```python
from build123d import *

# Parameters (mm, degrees)
SKETCH004_W  = 65.024
SKETCH004_H  = 49.2125
PAD004_DEPTH = 2.54
SKETCH005_W  = 49.341553
SKETCH005_H  = 34.925
PAD005_DEPTH = 2.54


with BuildPart() as inverterlowerbracket:
    # Sketch004 → Pad004 (new body)
    with BuildSketch(Plane.YZ):
        with Locations((-55.960957, 1378.268994)):
            Rectangle(SKETCH004_W, SKETCH004_H)
        with BuildLine():
            ThreePointArc((-82.122957, 1396.525244), (-85.297957, 1393.350244), (-82.122957, 1390.175244))
            Line((-82.122957, 1390.175244), (-59.897957, 1390.175244))
            ThreePointArc((-59.897957, 1390.175244), (-56.722957, 1393.350244), (-59.897957, 1396.525244))
            Line((-82.122957, 1396.525244), (-59.897957, 1396.525244))
        make_face(mode=Mode.SUBTRACT)
        with BuildLine():
            ThreePointArc((-82.122957, 1366.362744), (-85.297957, 1363.187744), (-82.122957, 1360.012744))
            Line((-82.122957, 1360.012744), (-59.897957, 1360.012744))
            ThreePointArc((-59.897957, 1360.012744), (-56.722957, 1363.187744), (-59.897957, 1366.362744))
            Line((-82.122957, 1366.362744), (-59.897957, 1366.362744))
        make_face(mode=Mode.SUBTRACT)
    extrude(amount=PAD004_DEPTH)

    # Sketch005 (on Face1 of Pad004) → Pad005 (join)
    with BuildSketch(Plane.ZX.offset(-23.448957)):
        with Locations((1378.334228, -14.922899)):
            Rectangle(SKETCH005_W, SKETCH005_H)
        with BuildLine():
            ThreePointArc((1364.309636, -11.747899), (1358.753386, -17.304149), (1364.309636, -22.860399))
            Line((1364.309636, -22.860399), (1390.105531, -22.860399))
            ThreePointArc((1390.105531, -22.860399), (1395.661781, -17.304149), (1390.105531, -11.747899))
            Line((1364.309636, -11.747899), (1390.105531, -11.747899))
        make_face(mode=Mode.SUBTRACT)
    extrude(amount=PAD005_DEPTH)


with BuildPart() as inverterlowerbracket_1:
    # Body003 placement: moved
    add(inverterlowerbracket.part.moved(Location((111.76, 19.05, 241.3))))


with BuildPart() as part_mirroring001:
    # Part__Mirroring001: instance of InverterLowerBracket
    add(inverterlowerbracket_1.part.mirror(Plane(origin=(0, 0, 0), x_dir=(0, -1, 0), z_dir=(1, 0, 0))))


with BuildPart() as part_mirroring001_1:
    # Part__Mirroring001 placement: moved
    add(part_mirroring001.part.moved(Location((749.3, 0, 0))))


solid = part_mirroring001_1.part
```
Work out the finished part from the listing and answer in its coordinate system (mm). A direction names the side the tool comes from. Give positions to 0.01 mm unless a question says otherwise; leave off trailing zeros. Loops run counter-clockwise (first coordinate to the right, second up) from the corner with the lowest first, then second, coordinate; pieces in that order, holes last. Notation, with made-up numbers: (45.25, 8.5) - (82.25, 8.5) arc R20 cw to (82.25, 15.5) - close; hole circle Ø11 at (8, 2). An arc over 180 degrees is marked (long way). Use CSV: the item, a comma, the result in double quotes. Start each with the question number.
(1) Determine the mould class of faces 1 (the face through (636.288, -37.674, 1634.58)), 2 (the face through (648, -1.859, 1619)), 3 (the face through (636, -37, 1594.963)) for opening direction Z: released by +Z, released by -Z, zero draft, split by the parting line, or undercut.
(2) Find section C-C, the plane x = 650.5. Determine the outline of the cut face in (y, z) (1 decimal).
(3) A tool of negligible diameter and unlimited length cuts with its end or side. For faces 4 (the face through (636.288, -66.247, 1604.558)), 5 (the face through (637.54, -37, 1620)), 6 (the face through (636, -37, 1644.175)), 7 (the face through (654.722, -3.147, 1600.055)), from which of +Z, -Z, +X, -X, +Y, -Y can it reach the whole face along a straight path? Write none if from no direction.
(4) Find section D-D, the plane z = 1635. Count the separate pieces of the cut face and the enclosed holes in it, plus the area to 3 significant figures.
(5) Find section B-B, the plane y = -45.5. Determine the outline of the cut face in (x, z), plus the area to 3 significant figures.
(6) Each of these flat-tipped pins is pushed along its axis until it touches: pin 1 (1.3 mm diameter, centred on x = 636, y = -33, fed in from +Z); pin 2 (12 mm diameter, centred on y = -22, z = 1623.5, fed in from +X). Where does it stop, or does it pass through?
(7) Find the intervals of material crossed by L1, parallel to X at y = -48.5, z = 1612.5; L2, parallel to Y at x = 649, z = 1608; L3, parallel to Y at x = 637, z = 1605.5, in increasing order.
Results found:
1,face 1,"undercut"
1,face 2,"zero draft"
1,face 3,"released by -Z"
2,outline,"(-4.4, 1595) - (-1.9, 1595) - (-1.9, 1602.1) - (-4.4, 1602.1) - close; (-4.4, 1634.9) - (-1.9, 1634.9) - (-1.9, 1644.3) - (-4.4, 1644.3) - close"
3,face 4,"+X, -X"
3,face 5,"+Z, -Z, +X, -Y"
3,face 6,"+Z, +X, -X, -Y"
3,face 7,"+Y, -Y"
4,separate pieces,"3"
4,enclosed holes,"0"
4,area,"160 mm^2"
5,outline,"(635, 1594.96) - (637.54, 1594.96) - (637.54, 1601.31) - (635, 1601.31) - close; (635, 1607.66) - (637.54, 1607.66) - (637.54, 1631.48) - (635, 1631.48) - close; (635, 1637.83) - (637.54, 1637.83) - (637.54, 1644.18) - (635, 1644.18) - close"
5,area,"92.7 mm^2"
6,pin 1,"z = 1644.18"
6,pin 2,"x = 637.54"
7,L1,"635 to 637.54"
7,L2,"-4.4 to -1.86"
7,L3,"-69.42 to -66.08, -37.84 to -1.86"
